Geometry check sheet. Reference: the model listing, model coordinates, mm. Face numbers are marked on the shaded views. A direction names the side the tool comes from. Round coordinates to 2 decimals unless told otherwise and drop trailing zeros. Order: outer loops, then holes, each group sorted by start corner. A loop starts at its lowest first (then second) coordinate and runs counter-clockwise, first axis right, second up. Notation, with made-up numbers: (34, 50.25) - (73, 50.25) arc R24 cw to (73, 66.25) - close; hole circle Ø9 at (-24, 52.5). An arc over 180 degrees is marked (long way). One line per question, with ' | ' between items. Start each with the question number.
Q1. Sectioned sample at A-A, the plane y = 0. Enter the section's corners in (x, z) (1 decimal).
Q2. Sectioned sample at C-C, the plane z = -14. Enter the section's corners in (x, y).
Q3. Tool access check on the marked faces 1 and 2. Record the directions out of +Z, -Z, +X, -X, +Y, -Y that give a thin tool (end or side, any length) a straight path to the whole face; none if there is none.
Q4. Gauge pin test, flat ends, axial feed: P1, Ø1.5, axis at x = -4, y = -0.5, coming from the -Z side; P2, Ø1.7, axis at y = 0, z = 13.49, coming from the -X side; P3, Ø1.5, axis at y = -1, z = 12, coming from the -X side; P4, Ø1.5, axis at x = -4, y = -9, coming from the -Z side. Record the tip position at first contact, or that the pin passes through.
Q5. Sectioned sample at D-D, the plane x = -0.75. Give the number of separate pieces and of enclosed holes in the cut face, then the cut area to 3 significant figures.
Q6. Material ranges on line 1 along Y through (x, z) = (-2.4, 0) (1 decimal); line 2 along Y through (x, z) = (-1.05, -0.5); line 3 along X through (y, z) = (-10, -9), recorded low to high.
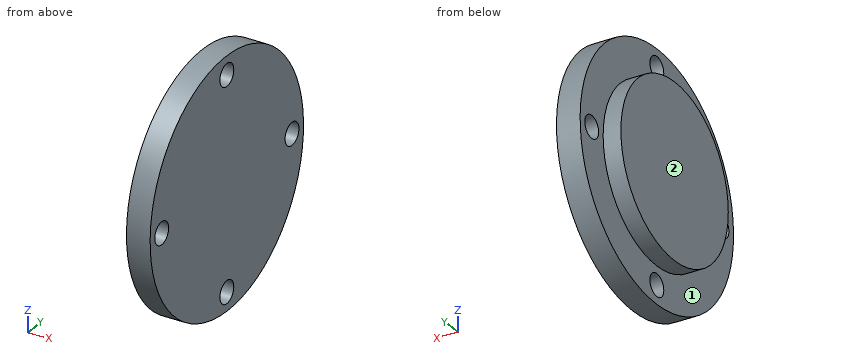
```python
from build123d import *

# Parameters (mm, degrees)
SKETCH2_R          = 1.4351
CUT_EXTRUDE1_DEPTH = 24.075588963


with BuildPart() as part:
    # Sketch1 → Revolve1 (revolve)
    with BuildSketch(Plane.XY, mode=Mode.PRIVATE) as revolve1_sk:
        Polygon((0, 0), (0, 15.875), (-3.048, 15.875), (-3.048, 11.1125), (-5.334, 11.1125), (-5.334, 0), align=None)
    revolve(revolve1_sk.sketch.rotate(Axis((0, 0, 0), (-1, 0, 0)), 90), axis=Axis((0, 0, 0), (-1, 0, 0)))

    # Sketch2 → Cut-Extrude1 (cut, through all)
    with BuildSketch(Plane(origin=(0, 0, 0), x_dir=(0, 0, -1), z_dir=(1, 0, 0))):
        with Locations((0, 13.4874)):
            Circle(SKETCH2_R)
        with Locations((13.4874, 0)):
            Circle(SKETCH2_R)
        with Locations((0, -13.4874)):
            Circle(SKETCH2_R)
        with Locations((-13.4874, 0)):
            Circle(SKETCH2_R)
    extrude(amount=-CUT_EXTRUDE1_DEPTH, mode=Mode.SUBTRACT)


solid = part.part
```
Determined:
1) outline: (-5.3, -11.1) - (-3, -11.1) - (-3, -12.1) - (0, -12.1) - (0, 12.1) - (-3, 12.1) - (-3, 11.1) - (-5.3, 11.1) - close; (-3, -15.9) - (0, -15.9) - (0, -14.9) - (-3, -14.9) - close; (-3, 14.9) - (0, 14.9) - (0, 15.9) - (-3, 15.9) - close
2) outline: (-3.05, -7.48) - (0, -7.48) - (0, -1.34) - (-3.05, -1.34) - close; (-3.05, 1.34) - (0, 1.34) - (0, 7.48) - (-3.05, 7.48) - close
3) face 1: -X | face 2: +Z, -Z, -X, +Y, -Y
4) P1: stops at z = -11.11 | P2: passes through | P3: stops at x = -3.05 | P4: stops at z = -7.44
5) separate pieces: 1 | enclosed holes: 4 | area: 766 mm2
6) line 1: y = -15.9 to -14.9, -12.1 to 12.1, 14.9 to 15.9 | line 2: y = -15.87 to -14.83, -12.14 to 12.14, 14.83 to 15.87 | line 3: x = -3.05 to 0
